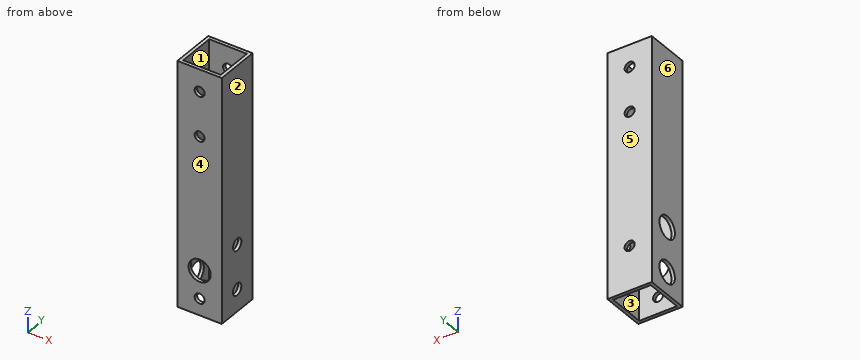
```python
from build123d import *

# Parameters (mm, degrees)
SKETCH_1_W          = 20
SKETCH_1_H          = 20
SKETCH_1_W_2        = 17
SKETCH_1_H_2        = 17
EXTRUDE_1_DEPTH     = 110
SKETCH_2_R          = 2.7
CUT_EXTRUDE_1_DEPTH = 25
SKETCH_3_R          = 2.25
CUT_EXTRUDE_2_DEPTH = 20
SKETCH_4_R          = 2.25
CUT_EXTRUDE_3_DEPTH = 5
SKETCH_5_R          = 5
CUT_EXTRUDE_4_DEPTH = 10
CUT_EXTRUDE_START   = -10
SKETCH_6_R          = 5
CUT_EXTRUDE_5_DEPTH = 10


with BuildPart() as part:
    # ｽｹｯﾁ1 → ﾎﾞｽ - 押し出し1 (new body)
    with BuildSketch(Plane.XY):
        Rectangle(SKETCH_1_W, SKETCH_1_H)
        Rectangle(SKETCH_1_W_2, SKETCH_1_H_2, mode=Mode.SUBTRACT)
    extrude(amount=EXTRUDE_1_DEPTH)

    # ｽｹｯﾁ2 → ｶｯﾄ - 押し出し1 (cut)
    with BuildSketch(Plane(origin=(10, 0, 0), x_dir=(0, 0, -1), z_dir=(1, 0, 0))):
        with Locations((-30, 0)):
            Circle(SKETCH_2_R)
        with Locations((-10, 0)):
            Circle(SKETCH_2_R)
    extrude(amount=-CUT_EXTRUDE_1_DEPTH, mode=Mode.SUBTRACT)

    # ｽｹｯﾁ3 → ｶｯﾄ - 押し出し2 (cut)
    with BuildSketch(Plane(origin=(0, 10, 0), x_dir=(1, 0, 0), z_dir=(0, 1, 0))):
        with Locations((0, -100)):
            Circle(SKETCH_3_R)
        with Locations((0, -80)):
            Circle(SKETCH_3_R)
        with Locations((0, -20)):
            Circle(SKETCH_3_R)
    extrude(amount=-CUT_EXTRUDE_2_DEPTH, mode=Mode.SUBTRACT)

    # ｽｹｯﾁ4 → ｶｯﾄ - 押し出し3 (cut)
    with BuildSketch(Plane(origin=(0, -10, 0), x_dir=(-1, 0, 0), z_dir=(0, -1, 0))):
        with Locations((0, -7.5)):
            Circle(SKETCH_4_R)
    extrude(amount=-CUT_EXTRUDE_3_DEPTH, mode=Mode.SUBTRACT)

    # ｽｹｯﾁ5 → ｶｯﾄ - 押し出し4 (cut)
    with BuildSketch(Plane(origin=(0, -10, 0), x_dir=(-1, 0, 0), z_dir=(0, -1, 0))):
        with Locations((0, -20)):
            Circle(SKETCH_5_R)
    extrude(amount=-CUT_EXTRUDE_4_DEPTH, mode=Mode.SUBTRACT)

    # ｽｹｯﾁ6 → ｶｯﾄ - 押し出し5 (cut)
    with BuildSketch(Plane(origin=(10, 0, 0), x_dir=(0, 0, -1), z_dir=(1, 0, 0)).offset(CUT_EXTRUDE_START)):
        with Locations((-10, 0)):
            Circle(SKETCH_6_R)
        with Locations((-30, 0)):
            Circle(SKETCH_6_R)
    extrude(amount=-CUT_EXTRUDE_5_DEPTH, mode=Mode.SUBTRACT)


solid = part.part
```
Input: part model. Units: mm. Frame: model coordinates. Face numbers are marked on the shaded views. A direction names the side the tool comes from. Coordinates: 2 decimals unless noted, no trailing zeros. Loops run counter-clockwise (first coordinate to the right, second up) from the corner with the lowest first, then second, coordinate; pieces in that order, holes last. Notation, with made-up numbers: (54, 15) -> (75, 15) arc R19 cw to (75, 22) -> close; hole circle Ø11 at (46, 73.5). An arc over 180 degrees is marked (long way). Use a Markdown table: item, result.
1) Cut plane A-A (z = 80). Return the cut outline in (x, y).
Results found:
| item | result |
|---|---|
| outline | (-10, -10) -> (-2.25, -10) -> (-2.25, -8.5) -> (-8.5, -8.5) -> (-8.5, 8.5) -> (-2.25, 8.5) -> (-2.25, 10) -> (-10, 10) -> close; (2.25, -10) -> (10, -10) -> (10, 10) -> (2.25, 10) -> (2.25, 8.5) -> (8.5, 8.5) -> (8.5, -8.5) -> (2.25, -8.5) -> close |
2) Cut plane B-B (z = 95.5). Return the cut outline in (x, y), then the cut area to 3 significant figures.
Results found:
| item | result |
|---|---|
| outline | (-10, -10) -> (10, -10) -> (10, 10) -> (-10, 10) -> close; hole (-8.5, -8.5) -> (8.5, -8.5) -> (8.5, 8.5) -> (-8.5, 8.5) -> close |
| area | 111 mm2 |
3) Material intervals for line 1 along Z through (x, y) = (0, 8.8); line 2 along Z through (x, y) = (0, -9.3); line 3 along Y through (x, z) = (-0.75, 46.5), sorted ascending. Write a range as from..to.
Results found:
| item | result |
|---|---|
| line 1 | z = 0..17.75, 22.25..77.75, 82.25..97.75, 102.25..110 |
| line 2 | z = 0..5.25, 9.75..15, 25..77.75, 82.25..97.75, 102.25..110 |
| line 3 | y = -10..-8.5, 8.5..10 |
4) Cut plane D-D (x = 0). Give the number of separate pieces and of enclosed holes in the cut face, then the cut area to 4 significant figures.
Results found:
| item | result |
|---|---|
| separate pieces | 9 |
| enclosed holes | 0 |
| area | 274.5 mm2 |
5) Cut plane C-C (z = 20). Return the cut outline in (x, y), then the cut area to 4 significant figures.
Results found:
| item | result |
|---|---|
| outline | (-10, -10) -> (-5, -10) -> (-5, -8.5) -> (-8.5, -8.5) -> (-8.5, 8.5) -> (-2.25, 8.5) -> (-2.25, 10) -> (-10, 10) -> close; (2.25, 8.5) -> (8.5, 8.5) -> (8.5, -8.5) -> (5, -8.5) -> (5, -10) -> (10, -10) -> (10, 10) -> (2.25, 10) -> close |
| area | 89.25 mm2 |
6) Contact query for flat-ended pins moving along their axis: pin 1 (3.5 mm diameter, centred on x = 0, z = 100, fed in from +Y); pin 2 (5 mm diameter, centred on x = 0, z = 20, fed in from -Y); pin 3 (6 mm diameter, centred on x = 6.5, y = -3.5, fed in from -Z). Output: stop coordinate, or through.
Results found:
| item | result |
|---|---|
| pin 1 | passes through |
| pin 2 | stops at y = 8.5 |
| pin 3 | stops at z = 0 |
7) Access query for the marked faces 1 and 2. Directions: +Z, -Z, +X, -X, +Y, -Y. A direction counts if a zero-diameter tool reaches every point of the face in a straight line with its end or side. Return the directions, or none.
Results found:
| item | result |
|---|---|
| face 1 | +Z, -Z |
| face 2 | +Z, -Z, +X, +Y, -Y |
8) Pull-direction query (Y, two-part tool) for the marked faces 3, 4, 5 and 6; classes: released by +Y, released by -Y, zero draft, split by the parting line, or undercut.
Results found:
| item | result |
|---|---|
| face 3 | undercut |
| face 4 | released by -Y |
| face 5 | released by +Y |
| face 6 | zero draft |
